from build123d import *

# Parameters (mm, degrees)
SKETCH2_W           = 25.4
SKETCH2_H           = 38.1
BOSS_EXTRUDE1_DEPTH = 6.35
SKETCH3_W           = 7.62
SKETCH3_H           = 7.62
BOSS_EXTRUDE2_DEPTH = 76.2
BOSS_EXTRUDE3_DEPTH = 7.62
FILLET1_R           = 2.54
SKETCH6_R           = 3.96875
CUT_EXTRUDE1_DEPTH  = 12.7
FILLET2_R           = 1.27


with BuildPart() as part:
    # Sketch2 → Boss-Extrude1 (new body)
    with BuildSketch(Plane(origin=(0, 0, 0), x_dir=(1, 0, 0), z_dir=(0, 1, 0))):
        with Locations((12.7, 19.05)):
            Rectangle(SKETCH2_W, SKETCH2_H)
    extrude(amount=BOSS_EXTRUDE1_DEPTH)

    # Sketch3 → Boss-Extrude2 (add)
    with BuildSketch(Plane(origin=(0, 6.35, 0), x_dir=(1, 0, 0), z_dir=(0, 1, 0))):
        with Locations((12.7, 26.67)):
            Rectangle(SKETCH3_W, SKETCH3_H)
    extrude(amount=BOSS_EXTRUDE2_DEPTH)

    # Sketch5 → Boss-Extrude3 (add)
    with BuildSketch(Plane.XY.offset(-22.86)):
        Polygon((3.175, 82.55), (22.225, 82.55), (22.225, 95.885), (19.05, 95.885), (19.05, 85.725), (6.35, 85.725), (6.35, 95.885), (3.175, 95.885), align=None)
    extrude(amount=-BOSS_EXTRUDE3_DEPTH)

    # Fillet1
    fillet1_edges = [part.edges().sort_by_distance(p)[0] for p in [
        (25.4, 6.35, -19.05),
        (8.89, 6.35, -26.67),
        (12.7, 6.35, -22.86),
        (12.7, 6.35, -38.1),
        (16.51, 6.35, -26.67),
        (12.7, 6.35, -30.48),
        (0, 6.35, -19.05),
        (12.7, 6.35, 0),
    ]]
    fillet(fillet1_edges, radius=FILLET1_R)

    # Sketch6 → Cut-Extrude1 (cut)
    with BuildSketch(Plane(origin=(0, 6.35, 0), x_dir=(1, 0, 0), z_dir=(0, 1, 0))):
        with Locations((12.7, 10.446236213)):
            Circle(SKETCH6_R)
    extrude(amount=-CUT_EXTRUDE1_DEPTH, mode=Mode.SUBTRACT)

    # Fillet2
    fillet2_edges = [part.edges().sort_by_distance(p)[0] for p in [
        (6.0325, 82.55, -30.48),
        (3.175, 89.2175, -30.48),
        (3.175, 82.55, -26.67),
        (22.225, 89.2175, -30.48),
        (19.3675, 82.55, -30.48),
        (22.225, 82.55, -26.67),
        (3.175, 89.2175, -22.86),
        (6.0325, 82.55, -22.86),
        (19.3675, 82.55, -22.86),
        (22.225, 89.2175, -22.86),
    ]]
    fillet(fillet2_edges, radius=FILLET2_R)


solid = part.part
Can you work these out from the model? Positions are in its coordinate system, mm. A direction names the side the tool comes from. Give positions to 0.01 mm unless a question says otherwise; leave off trailing zeros. Order: outer loops, then holes, each group sorted by start corner. A loop starts at its lowest first (then second) coordinate and runs counter-clockwise, first axis right, second up. Notation, with made-up numbers: M 82.25,-16.5 L 110.25,-16.5 A15 cw 110.25,-1.5 Z; hole C 85.5,19.5 d5. An arc over 180 degrees is marked long. One line per item, written item: value.
Item 1: If we section it at A-A on x = 12.7: Write out the boundary of the cut face in (y, z) (3 decimals), and give its area (3 significant figures).
Verdict:
outline: M 0,-38.1 L 3.81,-38.1 A2.54 ccw 6.35,-35.56 L 6.35,-33.02 A2.54 cw 8.89,-30.48 L 85.725,-30.48 L 85.725,-22.86 L 8.89,-22.86 A2.54 cw 6.35,-20.32 L 6.35,-14.415 L 0,-14.415 Z; M 0,-6.477 L 6.35,-6.477 L 6.35,-2.54 A2.54 ccw 3.81,0 L 0,0 Z
area: 796 mm2
Item 2: For pin 1 (13 mm diameter, centred on x = 10, y = 69, fed in from -Z); pin 2 (10 mm diameter, centred on x = 9, y = 18, fed in from +Z); pin 3 (10 mm diameter, centred on x = 7.5, z = -14.5, fed in from -Y); pin 4 (12.5 mm diameter, centred on x = 12.7, z = -10.45, fed in from +Y), each with a flat end and sliding along its axis, tell me the tip position at first contact or that it passes through.
Verdict:
pin 1: z = -30.48
pin 2: z = -22.86
pin 3: y = 0
pin 4: y = 6.35
Item 3: If we section it at B-B on z = -25.5: Write out the boundary of the cut face in (x, y) (3 decimals), and give its area (3 significant figures).
Verdict:
outline: M 0,0 L 25.4,0 L 25.4,3.81 A2.54 ccw 22.86,6.35 L 19.05,6.35 A2.54 cw 16.51,8.89 L 16.51,82.55 L 20.955,82.55 A1.27 ccw 22.225,83.82 L 22.225,95.885 L 19.05,95.885 L 19.05,85.725 L 6.35,85.725 L 6.35,95.885 L 3.175,95.885 L 3.175,83.82 A1.27 ccw 4.445,82.55 L 8.89,82.55 L 8.89,8.89 A2.54 cw 6.35,6.35 L 2.54,6.35 A2.54 ccw 0,3.81 Z
area: 866 mm2
Item 4: For faces 5 (the face through (13, 53, -30.48)), 6 (the face through (13, 53, -22.86)), 7 (the face through (7, 82.55, -27)), 8 (the face through (13, 85.725, -27)), which set-ups out of +Z, -Z, +X, -X, +Y, -Y let a thin tool reach every point of the face, with its end or its side?
Verdict:
face 5: -Z, +X, -X, +Y
face 6: +Z, +X, -X, +Y
face 7: +Z, -Z, -X
face 8: +Z, -Z, +Y
Item 5: If we section it at C-C on y = 12.5: Write out the boundary of the cut face in (x, z).
Verdict:
outline: M 8.89,-30.48 L 16.51,-30.48 L 16.51,-22.86 L 8.89,-22.86 Z
Item 6: If we mould it in two halves opening along Y, with no side actions, what happens to faces 1 (the face through (22.225, 90, -27)), 2 (the face through (17.62, 6.79, -26.76)), 3 (the face through (13, 0, -19)), 4 (the face through (12.878, 5.626, -37.336))? For each: pulls with the +Y half, pulls with the -Y half, needs draft (parallel to the pull), parting line crosses it, or undercut.
Verdict:
face 1: needs draft
face 2: undercut
face 3: pulls with the -Y half
face 4: pulls with the +Y half
Item 7: Please list where these lines run through material, in increasing order: line 1 (Y direction, x = 19.5, z = -29) (3 decimals); line 2 (Z direction, x = 12.7, y = 4.75); line 3 (Y direction, x = 22.75, z = -12.5).
Verdict:
line 1: 0 to 6.35, 82.55 to 95.885
line 2: -37.92 to -14.41, -6.48 to -0.18
line 3: 0 to 6.35
